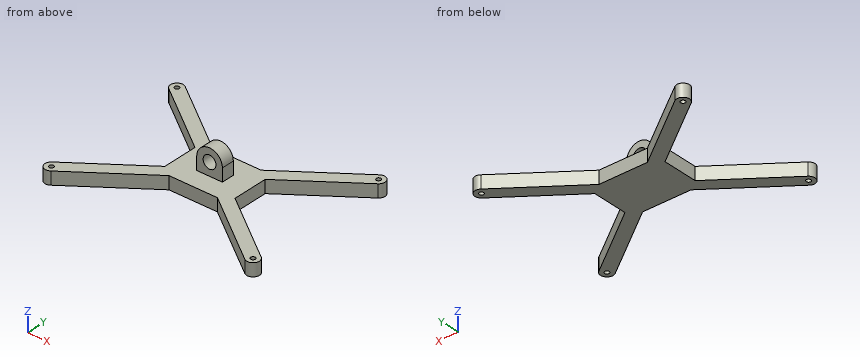
from build123d import *

# Parameters (mm, degrees)
ESQUISSE1_R        = 1.75
BOSS_EXTRU_1_DEPTH = 10
BOSS_EXTRU_3_START = 15
ESQUISSE4_R        = 5
BOSS_EXTRU_3_DEPTH = 10


with BuildPart() as part:
    # Esquisse1 → Boss.-Extru.1 (new body)
    with BuildSketch(Plane.XY):
        with BuildLine():
            Line((-2.952917385, 110.865117237), (51.171888599, 71.254033112))
            Line((51.171888599, 71.254033112), (51.171888599, 43.645966888))
            Line((51.171888599, 43.645966888), (-2.952917385, 4.034882763))
            ThreePointArc((-2.952917385, 4.034882763), (-4.034882763, -2.952917385), (2.952917385, -4.034882763))
            Line((2.952917385, -4.034882763), (59.638092267, 37.45))
            Line((59.638092267, 37.45), (97.361907733, 37.45))
            Line((97.361907733, 37.45), (154.047082615, -4.034882763))
            ThreePointArc((154.047082615, -4.034882763), (161.034882763, -2.952917385), (159.952917385, 4.034882763))
            Line((159.952917385, 4.034882763), (105.828111401, 43.645966888))
            Line((105.828111401, 43.645966888), (105.828111401, 71.254033112))
            Line((105.828111401, 71.254033112), (159.952917385, 110.865117237))
            ThreePointArc((159.952917385, 110.865117237), (161.034882763, 117.852917385), (154.047082615, 118.934882763))
            Line((154.047082615, 118.934882763), (97.361907733, 77.45))
            Line((97.361907733, 77.45), (59.638092267, 77.45))
            Line((59.638092267, 77.45), (2.952917385, 118.934882763))
            ThreePointArc((2.952917385, 118.934882763), (-4.034882763, 117.852917385), (-2.952917385, 110.865117237))
        make_face()
        Circle(ESQUISSE1_R, mode=Mode.SUBTRACT)
        with Locations((0, 114.9)):
            Circle(ESQUISSE1_R, mode=Mode.SUBTRACT)
        with Locations((157, 0)):
            Circle(ESQUISSE1_R, mode=Mode.SUBTRACT)
        with Locations((157, 114.9)):
            Circle(ESQUISSE1_R, mode=Mode.SUBTRACT)
    extrude(amount=BOSS_EXTRU_1_DEPTH)

    # Esquisse4 → Boss.-Extru.3 (add)
    with BuildSketch(Plane(origin=(0, 37.45, 123.316242038), x_dir=(1, 0, 0), z_dir=(0, 1, 0)).offset(BOSS_EXTRU_3_START)):
        with BuildLine():
            Line((88.5, 113.316242038), (88.5, 103.316242038))
            ThreePointArc((88.5, 103.316242038), (78.5, 93.316242038), (68.5, 103.316242038))
            Line((68.5, 103.316242038), (68.5, 113.316242038))
            Line((68.5, 113.316242038), (88.5, 113.316242038))
        make_face()
        with Locations((78.5, 103.316242038)):
            Circle(ESQUISSE4_R, mode=Mode.SUBTRACT)
    extrude(amount=BOSS_EXTRU_3_DEPTH)


solid = part.part
Can you work these out from the model? Positions are in its coordinate system, mm. Give positions to 0.01 mm unless a question says otherwise; leave off trailing zeros. Loops run counter-clockwise (first coordinate to the right, second up) from the corner with the lowest first, then second, coordinate; pieces in that order, holes last. Notation, with made-up numbers: (-6.75, 36.25) -> (30.25, 36.25) arc R11 ccw to (30.25, 48.25) -> close; hole circle Ø9 at (-12, -16). An arc over 180 degrees is marked (long way). Write item = value, one per line.
1) Suppose I cut it at B-B on z = 4. Write out the boundary of the cut face in (x, y).
Check result:
outline = (-2.95, 4.03) arc R5 ccw to (2.95, -4.03) -> (59.64, 37.45) -> (97.36, 37.45) -> (154.05, -4.03) arc R5 ccw to (159.95, 4.03) -> (105.83, 43.65) -> (105.83, 71.25) -> (159.95, 110.87) arc R5 ccw to (154.05, 118.93) -> (97.36, 77.45) -> (59.64, 77.45) -> (2.95, 118.93) arc R5 ccw to (-2.95, 110.87) -> (51.17, 71.25) -> (51.17, 43.65) -> close; hole circle Ø3.5 at (0, 0); hole circle Ø3.5 at (0, 114.9); hole circle Ø3.5 at (157, 0); hole circle Ø3.5 at (157, 114.9)
2) Suppose I cut it at D-D on z = 18.25. Write out the boundary of the cut face in (x, y).
Check result:
outline = (68.5, 52.45) -> (73.82, 52.45) -> (73.82, 62.45) -> (68.5, 62.45) -> close; (83.18, 52.45) -> (88.5, 52.45) -> (88.5, 62.45) -> (83.18, 62.45) -> close
3) Suppose I cut it at C-C on x = 0. Write out the boundary of the cut face in (y, z).
Check result:
outline = (-5, 0) -> (-1.75, 0) -> (-1.75, 10) -> (-5, 10) -> close; (1.75, 0) -> (6.2, 0) -> (6.2, 10) -> (1.75, 10) -> close; (108.7, 0) -> (113.15, 0) -> (113.15, 10) -> (108.7, 10) -> close; (116.65, 0) -> (119.9, 0) -> (119.9, 10) -> (116.65, 10) -> close
4) Suppose I cut it at A-A on x = 78.5. Write out the boundary of the cut face in (y, z).
Check result:
outline = (37.45, 0) -> (77.45, 0) -> (77.45, 10) -> (62.45, 10) -> (62.45, 15) -> (52.45, 15) -> (52.45, 10) -> (37.45, 10) -> close; (52.45, 25) -> (62.45, 25) -> (62.45, 30) -> (52.45, 30) -> close
5) Will these pins go through, and if not, where does the flat tip stop? pin 1 (4.5 mm diameter, centred on x = 0, y = 0, fed in from -Z); pin 2 (6 mm diameter, centred on y = 27.5, z = 5.5, fed in from -X); pin 3 (2 mm diameter, centred on y = 9.5, z = 6, fed in from -X); pin 4 (1.5 mm diameter, centred on y = 53, z = 18, fed in from +X).
Check result:
pin_1 = 0
pin_2 = 25.01
pin_3 = 3.15
pin_4 = 88.5
6) I need wall thicknesses on L1, parallel to X at y = 56, z = 20; L2, parallel to X at y = 114.9, z = 4; L3, parallel to Y at x = 157, z = 4.5. Which ranges of each line are inside material? Lowest first, please. Write a range as from..to.
Check result:
L1 = 68.5..73.5, 83.5..88.5
L2 = -5..-1.75, 1.75..8.47, 148.53..155.25, 158.75..162
L3 = -5..-1.75, 1.75..6.2, 108.7..113.15, 116.65..119.9
